Work out the finished part from the listing and answer in its coordinate system (mm). A direction names the side the tool comes from. Give positions to 0.01 mm unless a question says otherwise; leave off trailing zeros. Loops run counter-clockwise (first coordinate to the right, second up) from the corner with the lowest first, then second, coordinate; pieces in that order, holes last.
Autodesk Inventor part; units mm, degrees
ref_plane "YZ Plane" through (0, 0, 0) normal (1, 0, 0) x (0, 1, 0)
ref_plane "XZ Plane" through (0, 0, 0) normal (0, 1, 0) x (-1, 0, 0)
ref_plane "XY Plane" through (0, 0, 0) normal (0, 0, 1) x (1, 0, 0)
sketch "Sketch1" plane through (0, 0, 0) normal (0, 0, 1) x (1, 0, 0)
  line L0 (70, 0) -> (70, 25.4)
  line L1 (0, 25.4) -> (0, 0)
  arc A0 (9.6891, 25.4) -> (60.3109, 25.4) centre (35, 38.5) ccw
  line L2 (70, 25.4) -> (60.3109, 25.4)
  line L3 (9.6891, 25.4) -> (0, 25.4)
  line L4 (0, 0) -> (6.35, 0)
  line L5 (6.35, 0) -> (6.35, -6.35)
  line L6 (6.35, -6.35) -> (19.05, -6.35)
  line L7 (19.05, -6.35) -> (19.05, 0)
  line L8 (70, 0) -> (63.65, 0)
  line L9 (63.65, 0) -> (63.65, -6.35)
  line L10 (63.65, -6.35) -> (50.95, -6.35)
  line L11 (50.95, -6.35) -> (50.95, 0)
  line L12 (0, 0) -> (6.35, 0)
  line L13 (19.05, 0) -> (50.95, 0)
  line L14 (63.65, 0) -> (70, 0)
  dimension "d1" = 25.4
  dimension "d6" = 6.35
  dimension "d7" = 12.7
  dimension "d8" = 6.35
  dimension "d9" = 6.35
  dimension "d10" = 12.7
extrude "Extrusion1" add sketch "Sketch1" along normal blind 5.5563
properties part number "auger_holder"
Q1. Section C-C on x = 65.5 is taken. Give the vertices of the cut face in (y, z).
Q2. Section A-A on y = -1.5 is taken. Give the vertices of the cut face in (x, z), plus the area to 3 significant figures.
Q3. Given pin 1 (3 mm diameter, centred on x = 68, z = 4, fed in from -Y); pin 2 (3 mm diameter, centred on y = -3.5, z = 3.5, fed in from -X); pin 3 (1.7 mm diameter, centred on y = -2.5, z = 3, fed in from +X), each flat-ended and moving along its own axis, determine where each tip first touches the part or whether it passes through.
Q4. Consider line 1 along X through (y, z) = (-0.5, 0.75); line 2 along X through (y, z) = (20.5, 3.4); line 3 along Y through (x, z) = (64, 5.35). Determine where each line is inside the solid, lowest interval first.
Q5. Section D-D on y = 11 is taken. Give the vertices of the cut face in (x, z), plus the area to 3 significant figures.
Q6. Which of the six approach directions +Z, -Z, +X, -X, +Y, -Y give full straight-line access (tool end or side, diameter ignored) to faces 1 (the face through (50.95, -3, 3)), 2 (the face through (6.35, -3, 3)), 3 (the face through (63.65, -3, 3)), 4 (the face through (34.5, 9.7, 0))?
Q7. Section B-B on z = 2.1 is taken. Give the vertices of the cut face in (x, y).
Check result:
1. outline: (0, 0) - (25.4, 0) - (25.4, 5.56) - (0, 5.56) - close
2. outline: (6.35, 0) - (19.05, 0) - (19.05, 5.56) - (6.35, 5.56) - close; (50.95, 0) - (63.65, 0) - (63.65, 5.56) - (50.95, 5.56) - close
2. area: 141 mm2
3. pin 1: stops at y = 0
3. pin 2: stops at x = 6.35
3. pin 3: stops at x = 63.65
4. line 1: x = 6.35 to 19.05, 50.95 to 63.65
4. line 2: x = 0 to 12.9, 57.1 to 70
4. line 3: y = 0 to 25.4
5. outline: (0, 0) - (27.52, 0) - (27.52, 5.56) - (0, 5.56) - close; (42.48, 0) - (70, 0) - (70, 5.56) - (42.48, 5.56) - close
5. area: 306 mm2
6. face 1: +Z, -Z, -Y
6. face 2: +Z, -Z, -X, -Y
6. face 3: +Z, -Z, +X, -Y
6. face 4: -Z, +X, -X, +Y, -Y
7. outline: (0, 0) - (6.35, 0) - (6.35, -6.35) - (19.05, -6.35) - (19.05, 0) - (50.95, 0) - (50.95, -6.35) - (63.65, -6.35) - (63.65, 0) - (70, 0) - (70, 25.4) - (60.31, 25.4) arc R28.5 cw to (9.69, 25.4) - (0, 25.4) - close
